Autodesk Inventor part; units mm, degrees
ref_plane "YZ Plane" through (0, 0, 0) normal (1, 0, 0) x (0, 1, 0)
ref_plane "XZ Plane" through (0, 0, 0) normal (0, 1, 0) x (-1, 0, 0)
ref_plane "XY Plane" through (0, 0, 0) normal (0, 0, 1) x (1, 0, 0)
sketch "Sketch1" plane through (0, 0, 0) normal (0, 1, 0) x (-1, 0, 0)
  line L0 (-11.5, -9.45) -> (11.5, -9.45)
  line L1 (11.5, -9.45) -> (11.5, 9.45)
  line L2 (11.5, 9.45) -> (-11.5, 9.45)
  line L3 (-11.5, 9.45) -> (-11.5, -9.45)
  line L4 (12.5, -10.45) -> (-12.5, -10.45)
  line L5 (-12.5, -10.45) -> (-12.5, 10.45)
  line L6 (-12.5, 10.45) -> (12.5, 10.45)
  line L7 (12.5, 10.45) -> (12.5, -10.45)
  point P0 (0, 0)
  dimension "d0" = 23
  dimension "d4" = 9.45
  dimension "d6" = 11.5
  dimension "d21" = 18.9
  dimension "d22" = 20.9
  dimension "d23" = 10.45
  dimension "d24" = 25
  dimension "d25" = 12.5
extrude "Extrusion1" add sketch "Sketch1" along normal blind 14
sketch "Sketch2" plane through (0, 0, 0) normal (0, -1, 0) x (1, 0, 0)
  line L0 (2.75, 2.75) -> (-2.75, 2.75)
  line L1 (-2.75, 2.75) -> (-2.75, -2.75)
  line L2 (-2.75, -2.75) -> (2.75, -2.75)
  line L3 (2.75, -2.75) -> (2.75, 2.75)
  line L4 (-12.5, -10.45) -> (-12.5, 10.45)
  line L5 (-12.5, 10.45) -> (12.5, 10.45)
  line L6 (-12.5, -10.45) -> (-12.5, 10.45)
  line L7 (12.5, -10.45) -> (-12.5, -10.45)
  line L8 (-12.5, 10.45) -> (12.5, 10.45)
  line L9 (12.5, 10.45) -> (12.5, -10.45)
  line L10 (12.5, -10.45) -> (-12.5, -10.45)
  line L11 (-12.5, -10.45) -> (-12.5, 10.45)
  point P0 (0, 0)
  dimension "d10" = 5.5
  dimension "d11" = 5.5
  dimension "d26" = 2.75
  dimension "d27" = 2.75
extrude "Extrusion2" add sketch "Sketch2" along normal blind 0.5
sketch "Sketch4" plane through (-12.5, 14, 10.45) normal (0, 0, 1) x (1, 0, 0)
  line L0 (25, -14.5) -> (0, -14.5)
  line L1 (12.5, -14.5) -> (12.5, -3.3) construction
  line L2 (0, 0) -> (0, -14.5)
  circle A0 centre (12.5, -3.3) radius 2.9
  line L3 (0, 0) -> (25, 0)
  line L4 (12.5, -3.3) -> (15.4, -3.3) construction
  line L5 (12.5, -3.3) -> (9.6, -3.3) construction
  line L6 (15.4, -3.3) -> (15.4, 0)
  line L7 (9.6, -3.3) -> (9.6, 0)
  point P0 (12.5, -14)
  dimension "d28" = 12.5
  dimension "d29" = 11.2
  dimension "d30" = 5.8
extrude "Extrusion4" cut sketch "Sketch4" against normal through all
equation "\"d11\" = d10"
properties part number "motor_holder#1"
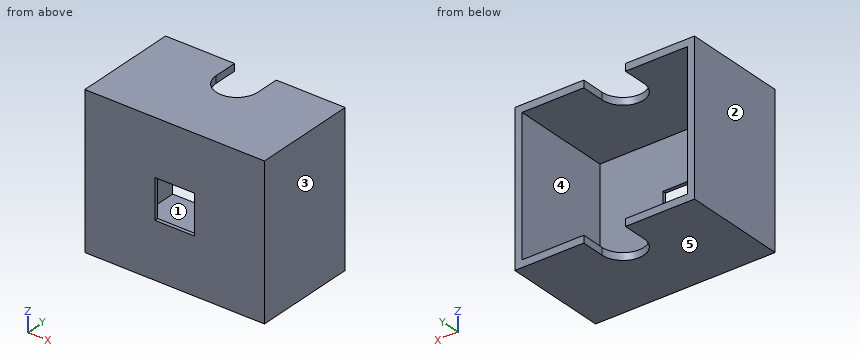
For this review, take the finished solid that the model builds, in its own axes (mm). Face numbers are marked on the shaded views. A direction names the side the tool comes from. Give positions to 0.01 mm unless a question says otherwise; leave off trailing zeros. Write each loop counter-clockwise with the first axis right and the second up, starting at its lowest first coordinate (ties: lowest second). Pieces come first, ordered by that corner, then holes. Notation, with made-up numbers: (-13, -3.75) -> (12, -3.75) arc R25 ccw to (12, 30.25) -> close; hole circle Ø5 at (17, 15.5). An arc over 180 degrees is marked (long way). Use CSV: the item, a comma, the result in double quotes.
Q1. Take a section at B-B, the plane x = 0. Write out the cut boundary in (y, z).
Conclusion:
outline,"(-0.5, -10.45) -> (7.8, -10.45) -> (7.8, -9.45) -> (0, -9.45) -> (0, -2.75) -> (-0.5, -2.75) -> close; (-0.5, 2.75) -> (0, 2.75) -> (0, 9.45) -> (7.8, 9.45) -> (7.8, 10.45) -> (-0.5, 10.45) -> close"
Q2. Tool access review of the marked faces 1 and 2: name each direction out of +Z, -Z, +X, -X, +Y, -Y from which nothing blocks a thin tool from reaching the whole face with its end or side.
Conclusion:
face 1,"+Y"
face 2,"+Z, -Z, -X, +Y, -Y"
Q3. To check wall thickness, follow probe 1 along Z at (x, y) = (-9, 13); probe 2 along X at (y, z) = (12.75, -3); probe 3 along Y at (x, z) = (4.5, -6). State the ranges of each line that lie inside material, in increasing order. Write a range as [from, to].
Conclusion:
probe 1,"[-10.45, -9.45], [9.45, 10.45]"
probe 2,"[-12.5, -11.5], [11.5, 12.5]"
probe 3,"[-0.5, 0]"
Q4. For P1, Ø5.5, axis at x = -4, z = 3, coming from the +Y side, flat-tipped, find the tip position at first contact; note if it passes through.
Conclusion:
P1,"y = 0"
Q5. Take a section at C-C, the plane z = 3.75. Write out the cut boundary in (x, y), then the cut area to 3 significant figures.
Conclusion:
outline,"(-12.5, -0.5) -> (12.5, -0.5) -> (12.5, 14) -> (11.5, 14) -> (11.5, 0) -> (-11.5, 0) -> (-11.5, 14) -> (-12.5, 14) -> close"
area,"40.5 mm2"
Q6. Mouldability with a two-part tool opening along X and no side actions: class the marked faces 3, 4 and 5 as pulls with the +X half, pulls with the -X half, needs draft (parallel to the pull), parting line crosses it, or undercut.
Conclusion:
face 3,"pulls with the +X half"
face 4,"undercut"
face 5,"needs draft"
Q7. Take a section at A-A, the plane y = 12.25. Write out the cut boundary in (x, z), then the cut area to 3 significant figures.
Conclusion:
outline,"(-12.5, -10.45) -> (-2.9, -10.45) -> (-2.9, -9.45) -> (-11.5, -9.45) -> (-11.5, 9.45) -> (-2.9, 9.45) -> (-2.9, 10.45) -> (-12.5, 10.45) -> close; (2.9, -10.45) -> (12.5, -10.45) -> (12.5, 10.45) -> (2.9, 10.45) -> (2.9, 9.45) -> (11.5, 9.45) -> (11.5, -9.45) -> (2.9, -9.45) -> close"
area,"76.2 mm2"
Q8. Take a section at D-D, the plane y = 7.25. Write out the cut boundary in (x, z).
Conclusion:
outline,"(-12.5, -10.45) -> (12.5, -10.45) -> (12.5, 10.45) -> (-12.5, 10.45) -> close; hole (-11.5, -9.45) -> (11.5, -9.45) -> (11.5, 9.45) -> (-11.5, 9.45) -> close"
